Read the model definition and answer for the solid it produces. Units are mm, in the model's axes. A direction names the side the tool comes from. Coordinates: 2 decimals unless noted, no trailing zeros. Order: outer loops, then holes, each group sorted by start corner. A loop starts at its lowest first (then second) coordinate and runs counter-clockwise, first axis right, second up.
```python
from build123d import *

# Parameters (mm, degrees)
SKETCH1_R           = 2.9972
SKETCH1_R_2         = 1.5875
SKETCH1_R_3         = 0.9271
BOSS_EXTRUDE1_DEPTH = 19.05
SKETCH2_R           = 2.5
CUT_EXTRUDE1_DEPTH  = 5


with BuildPart() as part:
    # Sketch1 → Boss-Extrude1 (new body)
    with BuildSketch(Plane.XY):
        with BuildLine():
            Line((0, 5.08), (8.89, 5.08))
            ThreePointArc((8.89, 5.08), (13.97, 0), (8.89, -5.08))
            Line((8.89, -5.08), (0, -5.08))
            ThreePointArc((0, -5.08), (-5.08, 0), (0, 5.08))
        make_face()
        with Locations(Location((0, 0, 0), (0, 0, 180))):
            Circle(SKETCH1_R, mode=Mode.SUBTRACT)
        with Locations(Location((8.89, 0, 0), (0, 0, 180))):
            Circle(SKETCH1_R_2, mode=Mode.SUBTRACT)
        with Locations(Location((4.445, -3.175, 0), (0, 0, 180))):
            Circle(SKETCH1_R_3, mode=Mode.SUBTRACT)
    extrude(amount=BOSS_EXTRUDE1_DEPTH)

    # Sketch2 → Cut-Extrude1 (cut)
    with BuildSketch(Plane.XY.offset(19.05)):
        with Locations((8.89, 0)):
            Circle(SKETCH2_R)
    extrude(amount=-CUT_EXTRUDE1_DEPTH, mode=Mode.SUBTRACT)

    # Sketch3 → Cut-Revolve1 (revolve, cut)
    with BuildSketch(Plane(origin=(0, 0, 0), x_dir=(1, 0, 0), z_dir=(0, 1, 0)), mode=Mode.PRIVATE) as cut_revolve1_sk:
        Polygon((11.39, -14.05), (10.4775, -13.501714685), (10.4775, -14.05), align=None)
    revolve(cut_revolve1_sk.sketch.rotate(Axis((8.89, 0, 14.05), (0, 0, 1)), 180), axis=Axis((8.89, 0, 14.05), (0, 0, 1)), mode=Mode.SUBTRACT)


solid = part.part
```
1) A cutting plane is placed at C-C, the plane x = -2.5. Determine the outline of the cut face in (y, z).
A:
outline: (-4.42, 0) - (-1.65, 0) - (-1.65, 19.05) - (-4.42, 19.05) - close; (1.65, 0) - (4.42, 0) - (4.42, 19.05) - (1.65, 19.05) - close
2) A cutting plane is placed at B-B, the plane z = 18.25. Determine the outline of the cut face in (x, y) (3 decimals), and give its area (3 significant figures).
A:
outline: (0, -5.08) - (8.89, -5.08) arc R5.08 ccw to (8.89, 5.08) - (0, 5.08) arc R5.08 ccw to start; hole circle Ø5.994 at (0, 0); hole circle Ø1.854 at (4.445, -3.175); hole circle Ø5 at (8.89, 0)
area: 121 mm2
3) Flat-ended cylindrical pins translate along their axes: pin 1 Ø1.9 at (x, y) = (8.89, 0) entering from +Z; pin 2 Ø3 at (y, z) = (2, 5.5) entering from +X. Find the tip coordinate at first contact, or state that the pin passes through.
A:
pin 1: passes through
pin 2: stops at x = 13.95
4) Which of the six approach directions +Z, -Z, +X, -X, +Y, -Y give full straight-line access (tool end or side, diameter ignored) to faces 4 (the cylindrical face through (-5.08, -0.11, 9.39)), 5 (the cylindrical face through (6.392, 0.11, 16.585))?
A:
face 4: +Z, -Z, -X
face 5: +Z
5) A cutting plane is placed at A-A, the plane y = 0. Determine the outline of the cut face in (x, z).
A:
outline: (-5.08, 0) - (-3, 0) - (-3, 19.05) - (-5.08, 19.05) - close; (3, 0) - (7.3, 0) - (7.3, 13.5) - (6.39, 14.05) - (6.39, 19.05) - (3, 19.05) - close; (10.48, 0) - (13.97, 0) - (13.97, 19.05) - (11.39, 19.05) - (11.39, 14.05) - (10.48, 13.5) - close
6) Determine the mould class of faces 1 (the flat face through (4, 5.08, 9)), 2 (the flat face through (5, -5.08, 9)), 3 (the cylindrical face through (5.13, -3.8, 9.39)) for opening direction Y: pulls with the +Y half, pulls with the -Y half, needs draft (parallel to the pull), parting line crosses it, or undercut.
A:
face 1: pulls with the +Y half
face 2: pulls with the -Y half
face 3: undercut
7) Straight lines are drawn through the part: line 1 (Y direction, x = 8.89, z = 16.5); line 2 (Y direction, x = 8.89, z = 4.5); line 3 (X direction, y = 1, z = 8.75). For each, find the intervals that lie inside material, in ascending order.
A:
line 1: y = -5.08 to -2.5, 2.5 to 5.08
line 2: y = -5.08 to -1.59, 1.59 to 5.08
line 3: x = -4.98 to -2.83, 2.83 to 7.66, 10.12 to 13.87
